Design review of the part built by this model. Coordinates are the model's own, in mm. Face numbers are marked on the shaded views. A direction names the side the tool comes from. Coordinates: 2 decimals unless noted, no trailing zeros. Loops run counter-clockwise (first coordinate to the right, second up) from the corner with the lowest first, then second, coordinate; pieces in that order, holes last. Notation, with made-up numbers: (24.25, -29) -> (72.25, -29) arc R21 ccw to (72.25, -5) -> close; hole circle Ø9 at (77.5, 89). An arc over 180 degrees is marked (long way). One line per item, written item: value. Start each with the question number.
1. Machinability: for the marked faces 1 and 2, which of the approach directions +Z, -Z, +X, -X, +Y, -Y give a long, thin tool a straight path to every point of the face, cutting with its end or side? Answer none if there is none.
2. For probe 1 along X at (y, z) = (0, -0.85); probe 2 along Y at (x, z) = (0.5, 8.5), list the stretches that pass through material, from the lowest coordinate up.
3. Add section C-C on z = -2.25. Write out the cut boundary in (x, y) (1 decimal).
4. Add section A-A on y = 0. Write out the cut boundary in (x, z) (1 decimal), plus the area to 3 significant figures.
5. Insertion check: pin 1 (2 mm diameter, centred on y = -6.5, z = -2.5, fed in from +X); pin 2 (2 mm diameter, centred on y = -5.5, z = 0.5, fed in from +X); pin 3 (6 mm diameter, centred on y = -7.5, z = 0, fed in from -X). Each pin has a flat end and moves straight along its axis. Give the tip position at first contact, or say it passes through.
6. Draft analysis for pull direction Y (two halves, no side actions). For the marked faces 3, 4 and 5, state which applies: pulls with the +Y half, pulls with the -Y half, needs draft (parallel to the pull), parting line crosses it, or undercut.
7. Add section D-D on z = 8.25. Write out the cut boundary in (x, y).
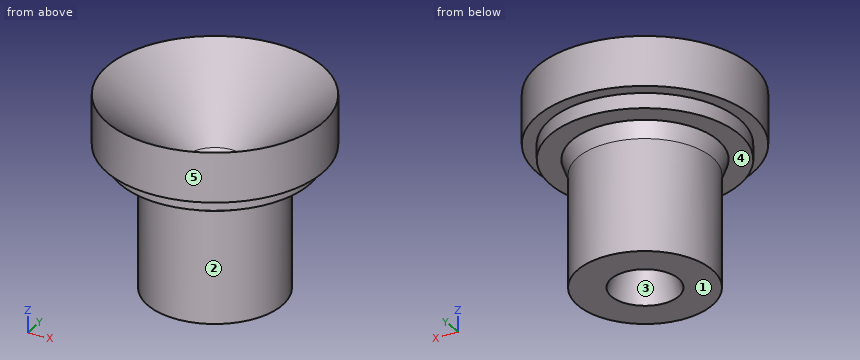
```python
from build123d import *


with BuildPart() as part:
    # Sketch2 → Revolve1 (revolve)
    with BuildSketch(Plane(origin=(0, 0, 0), x_dir=(0, 0, -1), z_dir=(1, 0, 0))):
        with BuildLine():
            Line((10.946291784, 7.9375), (-2.210908216, 7.9375))
            Line((-2.210908216, 7.9375), (-4.039708216, 8.62311403))
            Line((-4.039708216, 8.62311403), (-4.039708216, 11.1633))
            Line((-4.039708216, 11.1633), (-5.817708216, 11.1633))
            Line((-5.817708216, 11.1633), (-5.817708216, 12.7))
            Line((-5.817708216, 12.7), (-11.659708216, 12.7))
            Line((-11.659708216, 12.7), (-3.593152451, 3.42739423))
            ThreePointArc((-3.593152451, 3.42739423), (-1.974177838, 2.219145534), (0, 1.7907))
            Line((0, 1.7907), (2.794, 1.7907))
            Line((2.794, 1.7907), (10.946291784, 3.9751))
            Line((10.946291784, 3.9751), (10.946291784, 7.9375))
        make_face()
    revolve(axis=Axis((0, 0, 0), (0, 0, 1)))


solid = part.part
```
Worked answers:
1. face 1: -Z, +X, -X, +Y, -Y
1. face 2: -Z
2. probe 1: x = -7.94 to -1.79, 1.79 to 7.94
2. probe 2: y = -12.69 to -9.05, 9.05 to 12.69
3. outline: circle Ø15.9 at (0, 0); hole circle Ø3.6 at (0, 0)
4. outline: (-12.7, 5.8) -> (-11.2, 5.8) -> (-11.2, 4) -> (-8.6, 4) -> (-7.9, 2.2) -> (-7.9, -10.9) -> (-4, -10.9) -> (-1.8, -2.8) -> (-1.8, 0) arc R4.8 ccw to (-3.4, 3.6) -> (-12.7, 11.7) -> close; (1.8, -2.8) -> (4, -10.9) -> (7.9, -10.9) -> (7.9, 2.2) -> (8.6, 4) -> (11.2, 4) -> (11.2, 5.8) -> (12.7, 5.8) -> (12.7, 11.7) -> (3.4, 3.6) arc R4.8 ccw to (1.8, 0) -> close
4. area: 224 mm²
5. pin 1: stops at x = 5.72
5. pin 2: stops at x = 6.54
5. pin 3: stops at x = -6.54
6. face 3: undercut
6. face 4: needs draft
6. face 5: parting line crosses it
7. outline: circle Ø25.4 at (0, 0); hole circle Ø17.56 at (0, 0)
